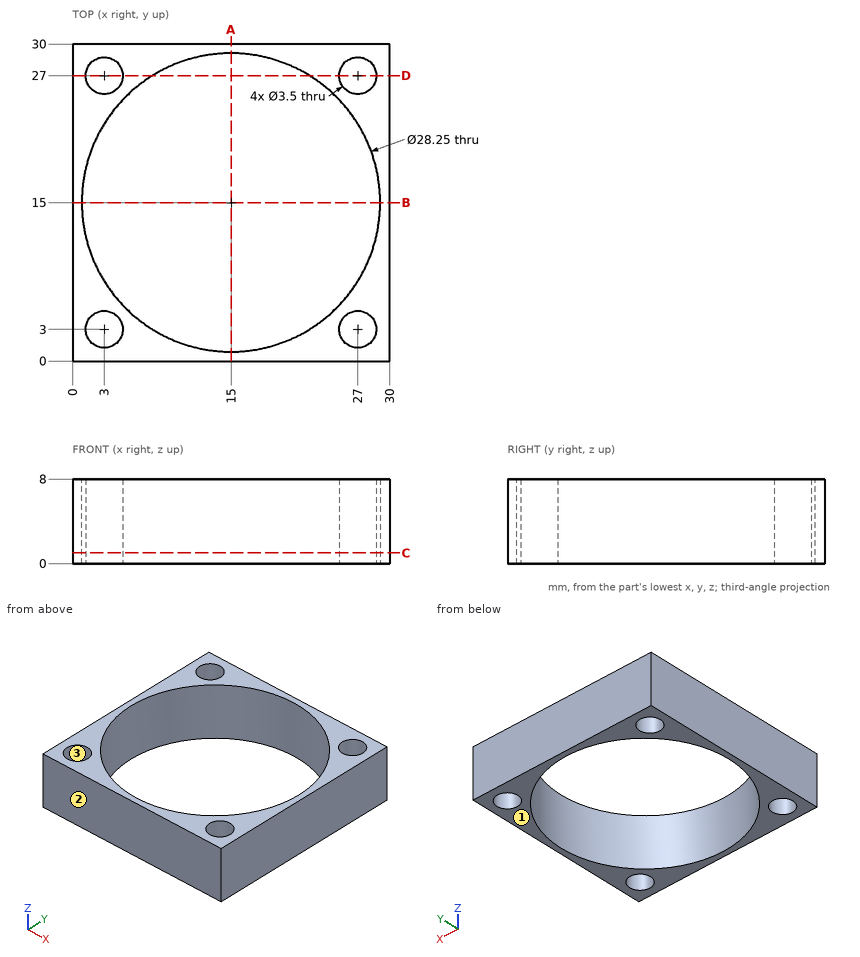
Geometry check sheet. Reference: drawing and pictorial views, mm from the part's lowest x, y, z. Coordinates: 2 decimals unless noted, no trailing zeros. Order: outer loops, then holes, each group sorted by start corner. A loop starts at its lowest first (then second) coordinate and runs counter-clockwise, first axis right, second up. Notation, with made-up numbers: (73.5, -36.5) -> (117.5, -36.5) arc R15 ccw to (117.5, -24.5) -> close; hole circle Ø8 at (53, 4). An arc over 180 degrees is marked (long way). Put each result on its own line as item: value. Start each with the question number.
1) Material ranges on L1, parallel to Y at x = 11.75, z = 2.5; L2, parallel to Y at x = 27, z = 3.25; L3, parallel to Y at x = 15, z = 2 (3 decimals), recorded low to high.
2) Cross-section at C-C (z = 1). Enter the section's corners in (x, y) (3 decimals), plus the area to 3 significant figures.
3) Cross-section at A-A (x = 15). Enter the section's corners in (y, z) (3 decimals).
4) Release check for a two-part mould opening along Y. For the marked faces 1, 2 and 3 record: pulls with the +Y half, pulls with the -Y half, needs draft (parallel to the pull), parting line crosses it, or undercut.
5) Cross-section at D-D (y = 27). Enter the section's corners in (x, z), plus the area to 3 significant figures.
Geometry check:
1. L1: y = 0 to 1.25, 28.75 to 30
1. L2: y = 0 to 1.25, 4.75 to 7.55, 22.45 to 25.25, 28.75 to 30
1. L3: y = 0 to 0.875, 29.125 to 30
2. outline: (0, 0) -> (30, 0) -> (30, 30) -> (0, 30) -> close; hole circle Ø28.25 at (15, 15); hole circle Ø3.5 at (3, 3); hole circle Ø3.5 at (3, 27); hole circle Ø3.5 at (27, 3); hole circle Ø3.5 at (27, 27)
2. area: 235 mm^2
3. outline: (0, 0) -> (0.875, 0) -> (0.875, 8) -> (0, 8) -> close; (29.125, 0) -> (30, 0) -> (30, 8) -> (29.125, 8) -> close
4. face 1: needs draft
4. face 2: pulls with the -Y half
4. face 3: undercut
5. outline: (0, 0) -> (1.25, 0) -> (1.25, 8) -> (0, 8) -> close; (4.75, 0) -> (7.55, 0) -> (7.55, 8) -> (4.75, 8) -> close; (22.45, 0) -> (25.25, 0) -> (25.25, 8) -> (22.45, 8) -> close; (28.75, 0) -> (30, 0) -> (30, 8) -> (28.75, 8) -> close
5. area: 64.8 mm^2
